The listing builds one solid part. Answer for the finished solid, in the listing's coordinates (mm). Face numbers are marked on the shaded views. A direction names the side the tool comes from. Give positions to 0.01 mm unless a question says otherwise; leave off trailing zeros. Write each loop counter-clockwise with the first axis right and the second up, starting at its lowest first coordinate (ties: lowest second). Pieces come first, ordered by that corner, then holes. Notation, with made-up numbers: (-20, 51) - (-5, 51) arc R22 ccw to (-5, 65) - close; hole circle Ø4 at (-31, -33.75). An arc over 180 degrees is marked (long way). Use a Markdown table: item, result. Add a question column.
from build123d import *

# Parameters (mm, degrees)
SKETCH_1_R               = 11
EXTRUDE_1_DEPTH          = 2
SKETCH_2_R               = 5
SKETCH_2_R_2             = 2.5
EXTRUDE_2_DEPTH          = 10
SKETCH_3_R               = 1.5
CUT_EXTRUDE_1_DEPTH      = 3
SKETCH_4_R               = 1.5
CUT_EXTRUDE_2_DEPTH      = 12
CUT_EXTRUDE_2_DEPTH_BACK = 12


with BuildPart() as part:
    # 草图1 → 凸台-拉伸1 (new body)
    with BuildSketch(Plane.XY):
        Circle(SKETCH_1_R)
    extrude(amount=EXTRUDE_1_DEPTH)

    # 草图2 → 凸台-拉伸2 (add)
    with BuildSketch(Plane.XY.offset(2)):
        Circle(SKETCH_2_R)
        Circle(SKETCH_2_R_2, mode=Mode.SUBTRACT)
    extrude(amount=EXTRUDE_2_DEPTH)

    # 草图3 → 切除-拉伸1 (cut, through all)
    with BuildSketch(Plane.XY.offset(2)):
        with Locations((0, 8)):
            Circle(SKETCH_3_R)
        with Locations((8, 0)):
            Circle(SKETCH_3_R)
        with Locations((0, -8)):
            Circle(SKETCH_3_R)
        with Locations((-8, 0)):
            Circle(SKETCH_3_R)
    extrude(amount=-CUT_EXTRUDE_1_DEPTH, mode=Mode.SUBTRACT)

    # 草图4 → 切除-拉伸2 (cut, two sides)
    with BuildSketch(Plane(origin=(0, 0, 0), x_dir=(0, 0, -1), z_dir=(1, 0, 0))) as cut_extrude_2_sk:
        with Locations((-7.289607981, 0)):
            Circle(SKETCH_4_R)
    extrude(amount=CUT_EXTRUDE_2_DEPTH, mode=Mode.SUBTRACT)
    extrude(cut_extrude_2_sk.sketch, amount=-CUT_EXTRUDE_2_DEPTH_BACK, mode=Mode.SUBTRACT)


solid = part.part
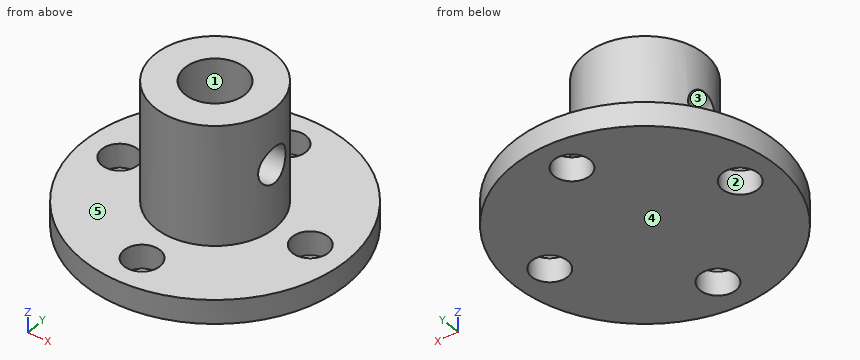
1. Consider L1, parallel to Y at x = -0.75, z = 1.5; L2, parallel to Y at x = 0, z = 0.95; L3, parallel to Y at x = 0, z = 6.25. Determine where each line is inside the solid, lowest interval first. Write a range as [from, to].
2. Which of the six approach directions +Z, -Z, +X, -X, +Y, -Y give full straight-line access (tool end or side, diameter ignored) to the marked faces 1 and 2?
3. The part is cut by section D-D (y = -8.75). Give the vertices of the cut face in (x, z).
4. Given P1, Ø4, axis at x = 0, y = -8, coming from the +Z side; P2, Ø1.5, axis at y = 5, z = 9, coming from the +X side; P3, Ø4, axis at x = -4, z = 5.5, coming from the -Y side, each flat-ended and moving along its own axis, determine where each tip first touches the part or whether it passes through.
5. For a pull along Z with two mould halves and no side action, classify the marked faces 3, 4 and 5 as released by +Z, released by -Z, zero draft, split by the parting line, or undercut.
6. The part is cut by section C-C (y = 0). Give the vertices of the cut face in (x, z).
7. The part is cut by section A-A (x = 0). Give the vertices of the cut face in (y, z), and give its area (3 significant figures).
8. The part is cut by section B-B (z = 6.5). Give the vertices of the cut face in (x, y).
Check values:
| question | item | result |
|---|---|---|
| 1 | L1 | y = [-10.97, -9.3], [-6.7, 6.7], [9.3, 10.97] |
| 1 | L2 | y = [-11, -9.5], [-6.5, 6.5], [9.5, 11] |
| 1 | L3 | y = [-5, -2.5], [2.5, 5] |
| 2 | face 1 | +Z |
| 2 | face 2 | +Z, -Z |
| 3 | outline | (-6.67, 0) - (-1.3, 0) - (-1.3, 2) - (-6.67, 2) - close; (1.3, 0) - (6.67, 0) - (6.67, 2) - (1.3, 2) - close |
| 4 | P1 | stops at z = 2 |
| 4 | P2 | stops at x = 2.63 |
| 4 | P3 | stops at y = -4.58 |
| 5 | face 3 | undercut |
| 5 | face 4 | released by -Z |
| 5 | face 5 | released by +Z |
| 6 | outline | (-11, 0) - (-9.5, 0) - (-9.5, 2) - (-11, 2) - close; (-6.5, 0) - (6.5, 0) - (6.5, 2) - (5, 2) - (5, 5.79) - (2.5, 5.79) - (2.5, 2) - (-2.5, 2) - (-2.5, 5.79) - (-5, 5.79) - (-5, 2) - (-6.5, 2) - close; (-5, 8.79) - (-2.5, 8.79) - (-2.5, 12) - (-5, 12) - close; (2.5, 8.79) - (5, 8.79) - (5, 12) - (2.5, 12) - close; (9.5, 0) - (11, 0) - (11, 2) - (9.5, 2) - close |
| 7 | outline | (-11, 0) - (-9.5, 0) - (-9.5, 2) - (-11, 2) - close; (-6.5, 0) - (6.5, 0) - (6.5, 2) - (5, 2) - (5, 12) - (2.5, 12) - (2.5, 2) - (-2.5, 2) - (-2.5, 12) - (-5, 12) - (-5, 2) - (-6.5, 2) - close; (9.5, 0) - (11, 0) - (11, 2) - (9.5, 2) - close |
| 7 | area | 82.0 mm2 |
| 8 | outline | (-4.83, -1.28) arc R5 ccw to (4.83, -1.28) - (2.15, -1.28) arc R2.5 cw to (-2.15, -1.28) - close; (-4.83, 1.28) - (-2.15, 1.28) arc R2.5 cw to (2.15, 1.28) - (4.83, 1.28) arc R5 ccw to start |
